Source: CAD feature listing. Evaluate the final solid. Frame: model axes, mm. A direction names the side the tool comes from. Give positions to 0.01 mm unless a question says otherwise; leave off trailing zeros. Write each loop counter-clockwise with the first axis right and the second up, starting at its lowest first coordinate (ties: lowest second). Pieces come first, ordered by that corner, then holes. Notation, with made-up numbers: (-18, 63) -> (3, 63) arc R3 ccw to (3, 68) -> close; hole circle Ø3 at (12, -25.5). An arc over 180 degrees is marked (long way). Write item = value, one per line.
from build123d import *

# Parameters (mm, degrees)
PAD004_DEPTH    = 2
SKETCH008_W     = 169
SKETCH008_H     = 61.7
PAD005_DEPTH    = 2
SKETCH009_R     = 2.2
POCKET002_DEPTH = 4.001
SKETCH012_W     = 159
SKETCH012_H     = 51.7
POCKET005_DEPTH = 2


with BuildPart() as part:
    # Sketch007 → Pad004 (new body)
    with BuildSketch(Plane.XZ):
        with BuildLine():
            Line((-2, 62.7), (-2, 0))
            ThreePointArc((-2, 0), (-1.414214, -1.414214), (0, -2))
            Line((0, -2), (170, -2))
            ThreePointArc((170, -2), (171.414214, -1.414214), (172, 0))
            Line((172, 0), (172, 62.7))
            ThreePointArc((172, 62.7), (171.414214, 64.114214), (170, 64.7))
            Line((170, 64.7), (0, 64.7))
            ThreePointArc((0, 64.7), (-1.414214, 64.114214), (-2, 62.7))
        make_face()
    extrude(amount=PAD004_DEPTH)

    # Sketch008 (on Face9 of Pad004) → Pad005 (join)
    with BuildSketch(Plane(origin=(0, 0, 0), x_dir=(1, 0, 0), z_dir=(0, 1, 0))):
        with Locations((85, -31.35)):
            Rectangle(SKETCH008_W, SKETCH008_H)
    extrude(amount=PAD005_DEPTH)

    # Sketch009 (on Face5 of Pad005) → Pocket002 (cut, through all)
    with BuildSketch(Plane.XZ.offset(2)):
        with Locations((2.5, 2.5)):
            Circle(SKETCH009_R)
        with Locations((2.5, 60.5)):
            Circle(SKETCH009_R)
        with Locations((167.5, 60.5)):
            Circle(SKETCH009_R)
        with Locations((167.5, 2.5)):
            Circle(SKETCH009_R)
    extrude(amount=-POCKET002_DEPTH, mode=Mode.SUBTRACT)

    # Sketch012 (on Face28 of Pocket002) → Pocket005 (cut)
    with BuildSketch(Plane(origin=(0, 2, 0), x_dir=(1, 0, 0), z_dir=(0, 1, 0))):
        with Locations((85, -31.35)):
            Rectangle(SKETCH012_W, SKETCH012_H)
    extrude(amount=-POCKET005_DEPTH, mode=Mode.SUBTRACT)


with BuildPart() as part_1:
    # Body003 placement: moved
    add(part.part.moved(Location((-5, -5, 0))))


solid = part_1.part
1) Cut plane A-A (x = 101). Return the cut outline in (y, z).
Computed:
outline = (-7, -2) -> (-5, -2) -> (-5, 0.5) -> (-3, 0.5) -> (-3, 5.5) -> (-5, 5.5) -> (-5, 57.2) -> (-3, 57.2) -> (-3, 62.2) -> (-5, 62.2) -> (-5, 64.7) -> (-7, 64.7) -> close
2) Material intervals for L1, parallel to X at y = -5.1, z = 60.5; L2, parallel to Z at x = 162.5, y = -6.05; L3, parallel to Z at x = 100, y = -4.1, sorted ascending.
Computed:
L1 = -7 to -4.7, -0.3 to 160.3, 164.7 to 167
L2 = -2 to 0.3, 4.7 to 58.3, 62.7 to 64.7
L3 = 0.5 to 5.5, 57.2 to 62.2
3) Cut plane B-B (z = 19). Return the cut outline in (x, y), then the cut area to 3 significant figures.
Computed:
outline = (-7, -7) -> (167, -7) -> (167, -5) -> (164.5, -5) -> (164.5, -3) -> (159.5, -3) -> (159.5, -5) -> (0.5, -5) -> (0.5, -3) -> (-4.5, -3) -> (-4.5, -5) -> (-7, -5) -> close
area = 368 mm²
4) Access query for faces 1 (the flat face through (79, -5, 31)), 2 (the flat face through (79, -7, 32)). Directions: +Z, -Z, +X, -X, +Y, -Y. A direction counts if a zero-diameter tool reaches every point of the face in a straight line with its end or side. Return the directions, or none.
Computed:
face_1 = +Y
face_2 = +Z, -Z, +X, -X, -Y
5) Contact query for flat-ended pins moving along their axis: pin 1 (1.6 mm diameter, centred on x = 115, y = -3.5, fed in from -Z); pin 2 (0.9 mm diameter, centred on y = -4, z = 1, fed in from +X); pin 3 (0.5 mm diameter, centred on y = -4, z = 1, fed in from -X); pin 4 (6 mm diameter, centred on x = 112.5, z = 54.5, fed in from +Y). Output: stop coordinate, or through.
Computed:
pin_1 = 0.5
pin_2 = 164.5
pin_3 = -4.5
pin_4 = -3
6) Draft query along X for faces 3 (the flat face through (80, -3, 59)), 4 (the cylindrical face through (-1.317, -5.028, 4.355)). Return one class per face: pulls with the +X half, pulls with the -X half, needs draft (parallel to the pull), parting line crosses it, or undercut.
Computed:
face_3 = needs draft
face_4 = undercut
